Check sheet for the modelled part. Datum: model origin and axes. Units: mm. Face numbers are marked on the shaded views. A direction names the side the tool comes from. Round coordinates to 2 decimals unless told otherwise and drop trailing zeros. Return JSON: item names as keys, results as strings.
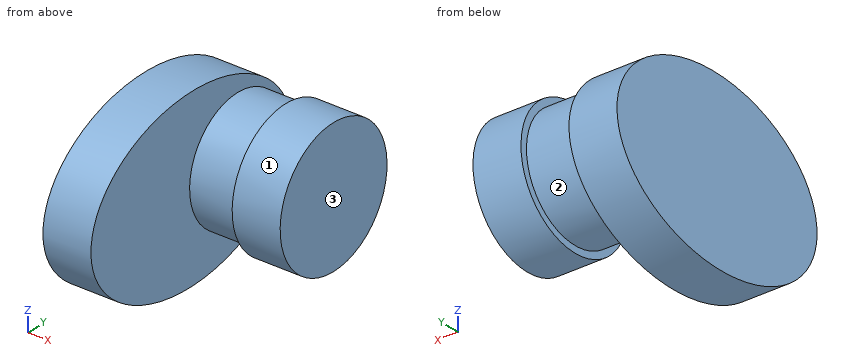
from build123d import *

# Parameters (mm, degrees)
SKETCH1_R           = 495.3
BOSS_EXTRUDE1_DEPTH = 355.6
SKETCH2_R           = 444.5
BOSS_EXTRUDE2_DEPTH = 355.6
SKETCH3_RX          = 927.1
SKETCH3_RY          = 647.7
BOSS_EXTRUDE3_DEPTH = 355.6


with BuildPart() as part:
    # Sketch1 → Boss-Extrude1 (new body)
    with BuildSketch(Plane(origin=(0, 0, 0), x_dir=(0, 0, -1), z_dir=(1, 0, 0))):
        Circle(SKETCH1_R)
    extrude(amount=-BOSS_EXTRUDE1_DEPTH)

    # Sketch2 → Boss-Extrude2 (add)
    with BuildSketch(Plane.ZY.offset(355.6)):
        Circle(SKETCH2_R)
    extrude(amount=BOSS_EXTRUDE2_DEPTH)

    # Sketch3 → Boss-Extrude3 (add)
    with BuildSketch(Plane.ZY.offset(711.2)):
        with Locations(Location((-9.638351828, -431.692416165), (0, 0, -91.279024431))):
            Ellipse(SKETCH3_RX, SKETCH3_RY)
    extrude(amount=BOSS_EXTRUDE3_DEPTH)


solid = part.part
Q1. Tool access check on the marked faces 1, 2 and 3. Record the directions out of +Z, -Z, +X, -X, +Y, -Y that give a thin tool (end or side, any length) a straight path to the whole face; none if there is none.
Results list:
{"face 1": "+X", "face 2": "none", "face 3": "+Z, -Z, +X, +Y, -Y"}
Q2. Material ranges on line 1 (X direction, y = -435, z = -215.5); line 2 (X direction, y = -1089, z = 331); line 3 (Z direction, x = -773.5, y = 67.5), recorded low to high.
Results list:
{"line 1": "-1066.8 to -711.2, -355.6 to 0", "line 2": "-1066.8 to -711.2", "line 3": "-549.77 to 541.9"}
Q3. Go/stop test with flat-tipped pins: pin 1 (12 mm diameter, centred on x = -919, z = -527.5, fed in from -Y); pin 2 (1 mm diameter, centred on x = -324, y = -99.5, fed in from -Z); pin 3 (2 mm diameter, centred on x = -846, y = -35, fed in from -Z). Record where each tip stops, or that it passes through.
Results list:
{"pin 1": "y = -1011.85", "pin 2": "z = -485.31", "pin 3": "z = -590.92"}
